Design review of the part built by this model. Coordinates are the model's own, in mm. A direction names the side the tool comes from. Give positions to 0.01 mm unless a question says otherwise; leave off trailing zeros. Order: outer loops, then holes, each group sorted by start corner. A loop starts at its lowest first (then second) coordinate and runs counter-clockwise, first axis right, second up. Notation, with made-up numbers: (26, 1.25) -> (40, 1.25) arc R20 cw to (40, 20.25) -> close; hole circle Ø9 at (75, 13). An arc over 180 degrees is marked (long way). Answer in a Markdown table with one row per item. Add a question column.
```python
from build123d import *

# Parameters (mm, degrees)
F0_W     = 119.480312
F0_H     = 94.520986
F0_W_2   = 100.755788
F0_H_2   = 74.011498
F1_DEPTH = 64.516
F2_W     = 60.856506
F2_H     = 10.254744
F3_DEPTH = 25.4
F4_R     = 18.095764
F5_DEPTH = 25.4
F6_R     = 18.255686
F7_DEPTH = 25.4


with BuildPart() as f1:
    # F0 (on Top) → F1 (new body)
    with BuildSketch(Plane.XY):
        Rectangle(F0_W, F0_H)
        Rectangle(F0_W_2, F0_H_2, mode=Mode.SUBTRACT)
    extrude(amount=F1_DEPTH)

    # F2 (on face) → F3 (cut)
    with BuildSketch(Plane.XY.offset(64.516)):
        with Locations((-1.609653, -42.133121)):
            Rectangle(F2_W, F2_H)
    extrude(amount=-F3_DEPTH, mode=Mode.SUBTRACT)

    # F4 (on face) → F5 (cut)
    with BuildSketch(Plane.YZ.offset(59.740156)):
        with Locations((0, 32.258)):
            Circle(F4_R)
    extrude(amount=-F5_DEPTH, mode=Mode.SUBTRACT)

    # F6 (on face) → F7 (cut)
    with BuildSketch(Plane(origin=(-59.740156, 0, 0), x_dir=(0, -1, 0), z_dir=(-1, 0, 0))):
        with Locations((0, 32.258)):
            Circle(F6_R)
    extrude(amount=-F7_DEPTH, mode=Mode.SUBTRACT)


solid = f1.part
```
1) Add section B-B, the plane x = -18. Write out the cut boundary in (y, z), and give its area (3 significant figures).
2) Add section C-C, the plane z = 20. Write out the cut boundary in (x, y).
3) Machinability: for faces 1 (the face through (-32.038, -42, 52)), 2 (the face through (-1, -47.26, 25)), 3 (the face through (-50.378, -17, 25)), 4 (the face through (-55.125, 2.377, 50.358)), 5 (the face through (59.74, -11, 17)), which of the approach directions +Z, -Z, +X, -X, +Y, -Y give a long, thin tool a straight path to every point of the face, cutting with its end or side? Answer none if there is none.
4) Mouldability with a two-part tool opening along X and no side actions: class faces 6 (the face through (4, 39, 64.516)), 7 (the face through (-59.74, -11, 17)), 8 (the face through (-2, -42, 39.116)) as +X half, -X half, draft (parallel to the pull), parting line (faces both ways), or undercut.
5) Add section A-A, the plane y = 29. Write out the cut boundary in (x, z).
6) Add section D-D, the plane y = 0. Write out the cut boundary in (x, z).
7) Clearance check with flat-ended pins moving along their axes: P1, Ø4, axis at x = -46.5, y = -29.5, coming from the +Z side; P2, Ø8, axis at x = -12, y = -44, coming from the +Z side. State where each tip first meets the part, or that it passes through.
8) For L1, parallel to X at y = -32, z = 18; L2, parallel to Y at x = -16, z = 23; L3, parallel to Z at x = 52.75, y = 0, list the stretches that pass through material, from the lowest coordinate up.
Verdict:
| question | item | result |
|---|---|---|
| 1 | outline | (-47.26, 0) -> (-37.01, 0) -> (-37.01, 39.12) -> (-47.26, 39.12) -> close; (37.01, 0) -> (47.26, 0) -> (47.26, 64.52) -> (37.01, 64.52) -> close |
| 1 | area | 1,060 mm2 |
| 2 | outline | (-59.74, -47.26) -> (59.74, -47.26) -> (59.74, -13.31) -> (50.38, -13.31) -> (50.38, -37.01) -> (-50.38, -37.01) -> (-50.38, -13.53) -> (-59.74, -13.53) -> close; (-59.74, 13.53) -> (-50.38, 13.53) -> (-50.38, 37.01) -> (50.38, 37.01) -> (50.38, 13.31) -> (59.74, 13.31) -> (59.74, 47.26) -> (-59.74, 47.26) -> close |
| 3 | face 1 | +Z, -Y |
| 3 | face 2 | +Z, -Z, +X, -X, -Y |
| 3 | face 3 | +Z, -Z |
| 3 | face 4 | -X |
| 3 | face 5 | +Z, -Z, +X, +Y, -Y |
| 4 | face 6 | draft |
| 4 | face 7 | -X half |
| 4 | face 8 | undercut |
| 5 | outline | (-59.74, 0) -> (-50.38, 0) -> (-50.38, 64.52) -> (-59.74, 64.52) -> close; (50.38, 0) -> (59.74, 0) -> (59.74, 64.52) -> (50.38, 64.52) -> close |
| 6 | outline | (-59.74, 0) -> (-50.38, 0) -> (-50.38, 14) -> (-59.74, 14) -> close; (-59.74, 50.51) -> (-50.38, 50.51) -> (-50.38, 64.52) -> (-59.74, 64.52) -> close; (50.38, 0) -> (59.74, 0) -> (59.74, 14.16) -> (50.38, 14.16) -> close; (50.38, 50.35) -> (59.74, 50.35) -> (59.74, 64.52) -> (50.38, 64.52) -> close |
| 7 | P1 | passes through |
| 7 | P2 | stops at z = 39.12 |
| 8 | L1 | x = -59.74 to -50.38, 50.38 to 59.74 |
| 8 | L2 | y = -47.26 to -37.01, 37.01 to 47.26 |
| 8 | L3 | z = 0 to 14.16, 50.35 to 64.52 |
